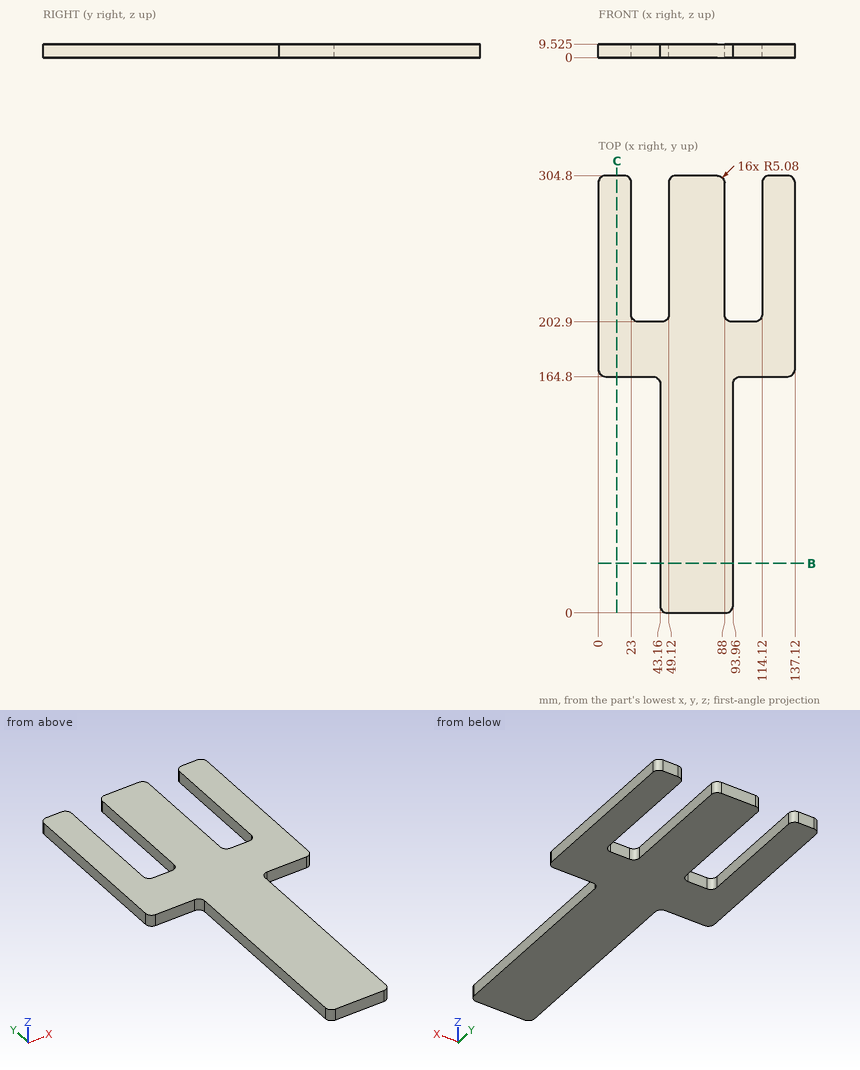
The drawing under review shows one solid part. Ordinate dimensions are in mm from its lowest x, y, z. Round coordinates to 2 decimals unless told otherwise and drop trailing zeros. Order: outer loops, then holes, each group sorted by start corner. A loop starts at its lowest first (then second) coordinate and runs counter-clockwise, first axis right, second up. Notation, with made-up numbers: (86.25, 54.5) - (94.25, 54.5) arc R11 cw to (94.25, 70.5) - close; hole circle Ø2 at (-15, 36.5). An arc over 180 degrees is marked (long way). Return JSON: item names as keys, results as strings.
Q1. Wall thickness on L1, parallel to X at y = 260, z = 5.5; L2, parallel to Y at x = 27.5, z = 6.5; L3, parallel to X at y = 18, z = 3: over which ranges is each line inside the solid? List them lowest first. Write a range as [from, to].
Computed values:
{"L1": "x = [0, 23], [49.12, 88], [114.12, 137.12]", "L2": "y = [164.8, 202.93]", "L3": "x = [43.16, 93.96]"}
Q2. Consider section B-B on y = 34.5. Write out the cut boundary in (x, z) (3 decimals), plus the area to 3 significant figures.
Computed values:
{"outline": "(43.16, 0) - (93.96, 0) - (93.96, 9.525) - (43.16, 9.525) - close", "area": "484 mm2"}
Q3. For pin 1 Ø5 at (y, z) = (47.5, 6.5) entering from -X; pin 2 Ø3 at (y, z) = (68, 4) entering from +X; pin 3 Ø1.5 at (x, z) = (107, 3.5) entering from +Y, all flat-tipped, find the tip position at first contact; note any pin that passes through.
Computed values:
{"pin 1": "stops at x = 43.16", "pin 2": "stops at x = 93.96", "pin 3": "stops at y = 202.9"}
Q4. Consider section C-C on x = 13. Write out the cut boundary in (y, z) (3 decimals), plus the area to 3 significant figures.
Computed values:
{"outline": "(164.8, 0) - (304.8, 0) - (304.8, 9.525) - (164.8, 9.525) - close", "area": "1,330 mm2"}
